Model file for the job. Use its own axes, mm. A direction names the side the tool comes from. Coordinates: 2 decimals unless noted, no trailing zeros. Write each loop counter-clockwise with the first axis right and the second up, starting at its lowest first coordinate (ties: lowest second). Pieces come first, ordered by that corner, then holes. Notation, with made-up numbers: M 35.25,-30 L 61.25,-30 A13 cw 61.25,-17 Z; hole C 88,17.5 d2. An arc over 180 degrees is marked long. Put each result on its own line as item: value. Start each with the question number.
Q1. Which spindle directions (+Z, -Z, +X, -X, +Y, -Y) get a long thin tool onto all of the face, cutting with end or side? Do faces 1 (the flat face through (168.67, -29.78, -10.04)), 2 (the flat face through (74, 127, 0)), 3 (the flat face through (151.88, -20.4, -8.21)). Say none if no direction does.
Q2. Drill centre lines: line 1 along Z through (x, y) = (79.5, 226); line 2 along Y through (x, z) = (65.5, -4.5); line 3 along Y through (x, z) = (36.5, -1). Where is each one in solid material? Low to high.
Q3. Pull direction X, two halves, no side cores. Call faces 4 (the flat face through (143.88, 2.45, 1.82)), 5 (the flat face through (194.79, -2.48, 20.86)), 6 (the flat face through (100, 250, 3)): pulls with the +X half, pulls with the -X half, needs draft (parallel to the pull), parting line crosses it, or undercut.
Q4. Cut at A-A (x = 177.5). Write the cut outline in (y, z), then the cut area to 3 significant figures.
Q5. Cut at C-C (x = 95). Write the cut outline in (y, z), then the cut area to 3 significant figures.
Q6. Drop flat-ended pins along their axis: pin 1 (2 mm diameter, centred on x = 162, z = 1, fed in from -Y); pin 2 (12 mm diameter, centred on y = 65.5, z = -9.5, fed in from -X) (3 decimals); pin 3 (12 mm diameter, centred on y = 96.5, z = 19, fed in from -X); pin 4 (22 mm diameter, centred on x = 178.5, z = 10, fed in from -Y). Give the stop position or say it passes through.
Q7. Cut at B-B (y = 108). Write the cut outline in (x, z), then the cut area to 3 significant figures.
```python
from build123d import *

# Parameters (mm, degrees)
F0_W      = 150
F0_H      = 250
F1_DEPTH  = 5
F3_DEPTH  = 150
F5_DEPTH  = 250
F7_W      = 58.9762479067
F7_H      = 46.3181659579
F8_DEPTH  = 3.61943
F9_W      = 66.3050051284
F9_H      = 23.7932279706
F10_DEPTH = 25
F11_W     = 9.7743958235
F11_H     = 36.3947637379
F12_DEPTH = 25
F13_W     = 91.9819101691
F13_H     = 53.4567786381
F14_DEPTH = 25
F17_DEPTH = 42.79442
F18_DEPTH = 37.25584


with BuildPart() as f1:
    # F0 (on Top) → F1 (new body)
    with BuildSketch(Plane.XY):
        with Locations((75, 125)):
            Rectangle(F0_W, F0_H)
    extrude(amount=F1_DEPTH)

    # F2 (on Right) → F3 (join)
    with BuildSketch(Plane.YZ):
        Polygon((-25.8566159755, -16.7061649263), (0, 0), (0, 5), (-27.978492185, -13.0771259965), align=None)
    extrude(amount=F3_DEPTH)

    # F4 (on Front) → F5 (join)
    with BuildSketch(Plane.XZ):
        Polygon((150, 5), (150, 0), (200, 20), (200, 25), align=None)
    extrude(amount=-F5_DEPTH)

    # F7 (on 3pt) → F8 (join)
    with BuildSketch(Plane(origin=(15.2143755699, 24.5753222078, -38.0359389247), x_dir=(0.9479297598, -0.1728350436, 0.2675018096), z_dir=(-0.3184794663, -0.5144302811, 0.7961986658))):
        with Locations((171.1452230811, -7.3043461889)):
            Rectangle(F7_W, F7_H)
    extrude(amount=F8_DEPTH)

    # F9 (on face) → F10 (cut)
    with BuildSketch(Plane(origin=(18.9655172414, 0, -47.4137931034), x_dir=(0.9284766909, 0, 0.3713906764), z_dir=(-0.3713906764, 0, 0.9284766909))):
        with Locations((174.2809595788, 11.8966139853)):
            Rectangle(F9_W, F9_H)
    extrude(amount=F10_DEPTH, mode=Mode.SUBTRACT)

    # F11 (on face) → F12 (cut)
    with BuildSketch(Plane.XY.offset(5)):
        with Locations((145.1128020883, 18.197381869)):
            Rectangle(F11_W, F11_H)
    extrude(amount=F12_DEPTH, mode=Mode.SUBTRACT)

    # F13 (on face) → F14 (cut)
    with BuildSketch(Plane.YZ.offset(200)):
        with Locations((-13.2915489376, 13.6362598278)):
            Rectangle(F13_W, F13_H)
    extrude(amount=F14_DEPTH, mode=Mode.SUBTRACT)

    # F16 (on face) → F17 (cut)
    with BuildSketch(Plane(origin=(121.6211489037, -89.4544048238, -10.2533341545), x_dir=(0.5890555913, 0.8065651439, -0.0496606377), z_dir=(0.8037140341, -0.5911452179, -0.0677575293))):
        Polygon((66.8091401458, 0), (89.8736044765, 14.5051842555), (116.4209321141, 42.6778681576), align=None)
    extrude(amount=F17_DEPTH, mode=Mode.SUBTRACT)

    # F18 (cut): a face of the model
    f18_faces = [f1.faces().sort_by_distance(p)[0] for p in [
        (175.9683447832, -17.0287264276, 2.5203105636),
    ]]
    extrude(f18_faces, amount=-F18_DEPTH, mode=Mode.SUBTRACT)


solid = f1.part
```
Computed values:
1. face 1: -Z, +X, -Y
1. face 2: -Z, +X, -X, +Y
1. face 3: none
2. line 1: 0 to 5
2. line 2: -14.7 to -6.96
2. line 3: -9.29 to -1.55
3. face 4: undercut
3. face 5: pulls with the -X half
3. face 6: needs draft
4. outline: M -31.71,-7.06 L -30.6,-8.77 L 0,11 L 250,11 L 250,16 L 1.88,16 L -18.23,-0.41 Z; M 0,15.62 L 0.59,16 L 0,16 Z
4. area: 1,300 mm2
5. outline: M -27.98,-13.08 L -25.86,-16.71 L 0,0 L 250,0 L 250,5 L 0,5 Z
5. area: 1,380 mm2
6. pin 1: y = -8.73
6. pin 2: through
6. pin 3: x = 170
6. pin 4: y = -21.28
7. outline: M 0,0 L 150,0 L 200,20 L 200,25 L 150,5 L 0,5 Z
7. area: 1,000 mm2
